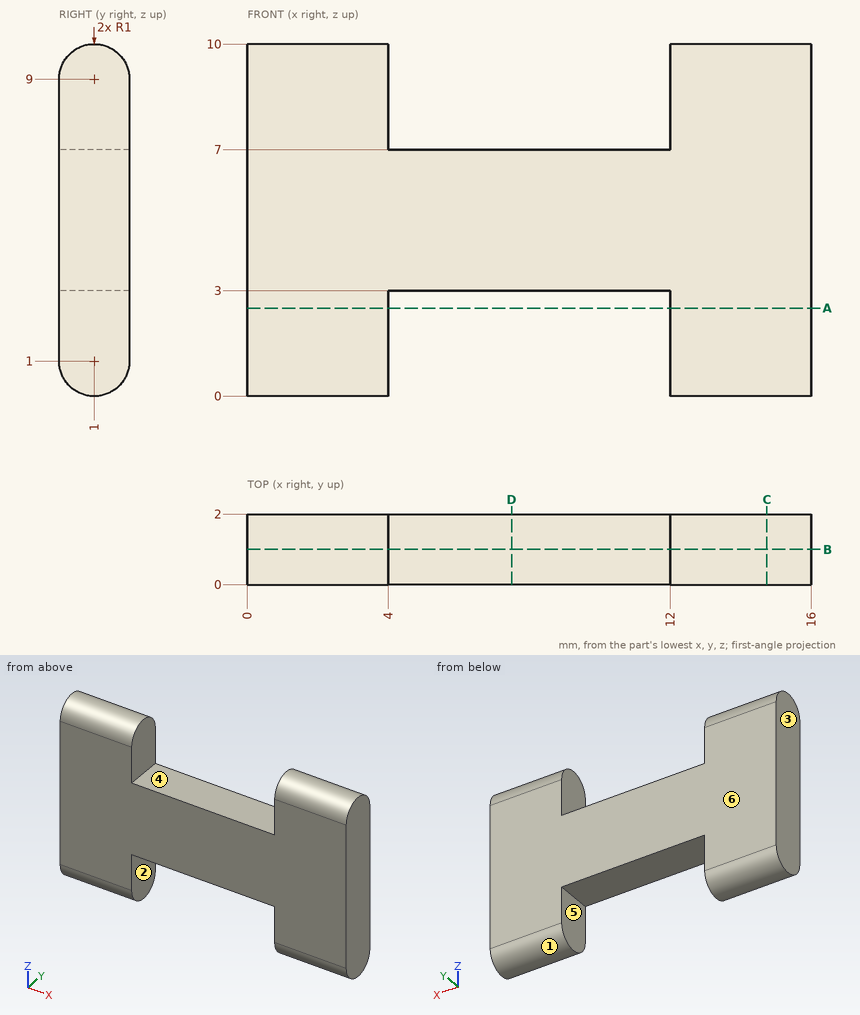
Job drawing, mm, ordinate dimensions from the low corner. One solid piece. A direction names the side the tool comes from. Round coordinates to 2 decimals unless told otherwise and drop trailing zeros. Order: outer loops, then holes, each group sorted by start corner. A loop starts at its lowest first (then second) coordinate and runs counter-clockwise, first axis right, second up. Notation, with made-up numbers: (71.5, -36.75) -> (82.5, -36.75) arc R13 cw to (82.5, -13.75) -> close; hole circle Ø6 at (25.5, 21). An arc over 180 degrees is marked (long way). Answer in a Markdown table with one row per item.
1) Wall check: L1, parallel to X at y = 1.7, z = 0.5; L2, parallel to Z at x = 6.25, y = 1.45; L3, parallel to Z at x = 2.25, y = 1.1. Give the ranges that are in metal, low to high.
Values:
| item | result |
|---|---|
| L1 | 0 to 4, 12 to 16 |
| L2 | 3 to 7 |
| L3 | 0.01 to 9.99 |
2) Pin check, flat tip, straight feed: P1, Ø1, axis at x = 8.5, y = 1, coming from the +Z side. Stop position of the tip, or through.
Values:
| item | result |
|---|---|
| P1 | z = 7 |
3) Mould opens along X. For the marked faces 1, 2 and 3 say: released by +X, released by -X, zero draft, split by the parting line, or undercut.
Values:
| item | result |
|---|---|
| face 1 | zero draft |
| face 2 | undercut |
| face 3 | released by -X |
4) Band-saw the part on C-C on x = 14.75. Give the cut face in (y, z), and give its area (3 significant figures).
Values:
| item | result |
|---|---|
| outline | (0, 1) arc R1 ccw to (2, 1) -> (2, 9) arc R1 ccw to (0, 9) -> close |
| area | 19.1 mm2 |
5) Which spindle directions (+Z, -Z, +X, -X, +Y, -Y) get a long thin tool onto all of the face, cutting with end or side? Do the marked faces 4, 5 and 6. Say none if no direction does.
Values:
| item | result |
|---|---|
| face 4 | +Z, +Y, -Y |
| face 5 | -Z, +Y, -Y |
| face 6 | +Z, -Z, +X, -X, +Y |
6) Band-saw the part on B-B on y = 1. Give the cut face in (x, z).
Values:
| item | result |
|---|---|
| outline | (0, 0) -> (4, 0) -> (4, 3) -> (12, 3) -> (12, 0) -> (16, 0) -> (16, 10) -> (12, 10) -> (12, 7) -> (4, 7) -> (4, 10) -> (0, 10) -> close |
7) Band-saw the part on D-D on x = 7.5. Give the cut face in (y, z).
Values:
| item | result |
|---|---|
| outline | (0, 3) -> (2, 3) -> (2, 7) -> (0, 7) -> close |
8) Band-saw the part on A-A on z = 2.5. Give the cut face in (x, y), and give its area (3 significant figures).
Values:
| item | result |
|---|---|
| outline | (0, 0) -> (4, 0) -> (4, 2) -> (0, 2) -> close; (12, 0) -> (16, 0) -> (16, 2) -> (12, 2) -> close |
| area | 16.0 mm2 |
